```python
from build123d import *

# Parameters (mm, degrees)
F0_W     = 19.05
F0_H     = 90.4875
F1_DEPTH = 304.8
F3_W     = 12.7
F3_H     = 101.6
F4_DEPTH = 12.7
F6_DEPTH = 304.8
F8_DEPTH = 304.8


with BuildPart() as f1:
    # F0 (on Front) → F1 (new body)
    with BuildSketch(Plane.XZ):
        with Locations((9.525, 45.24375)):
            Rectangle(F0_W, F0_H)
    extrude(amount=F1_DEPTH)

    # F3 (on offset) → F4 (cut)
    with BuildSketch(Plane.XZ.offset(25.4)):
        with Locations((-1.8542, 50.8)):
            Rectangle(F3_W, F3_H)
    extrude(amount=-F4_DEPTH, mode=Mode.SUBTRACT)

    # F5 (on Front) → F6 (cut)
    with BuildSketch(Plane.XZ):
        Polygon((-2.3876, -5.089026), (26.1874, -5.089026), (26.1874, 0), (16.6624, 0), (15.604067, 4.7625), (12.429067, 4.7625), (11.370733, 0), (8.195733, 0), (7.1374, 4.7625), (-2.3876, 4.7625), align=None)
    extrude(amount=F6_DEPTH, mode=Mode.SUBTRACT)

    # F7 (on Front) → F8 (cut)
    with BuildSketch(Plane.XZ):
        Polygon((26.1874, 90.4875), (26.1874, 95.576526), (-2.3876, 95.576526), (-2.3876, 85.725), (7.1374, 85.725), (8.195733, 90.4875), (11.370733, 90.4875), (12.429067, 85.725), (15.604067, 85.725), (16.6624, 90.4875), align=None)
    extrude(amount=F8_DEPTH, mode=Mode.SUBTRACT)


solid = f1.part
```
The model under review builds one solid part; all positions refer to its coordinate system, in mm. A direction names the side the tool comes from. Round coordinates to 2 decimals unless told otherwise and drop trailing zeros. Answer as a JSON object with one key per item and string values. Group by question number.
1) For line 1 (X direction, y = -232, z = 86); line 2 (Z direction, x = 14, y = -103) (1 decimal); line 3 (X direction, y = -87.5, z = 86.5), list the stretches that pass through material, from the lowest coordinate up. Write a range as [from, to].
2) For pin 1 Ø5 at (x, y) = (4.5, -273) entering from -Z; pin 2 Ø1.6 at (x, y) = (13.5, -149.5) entering from +Z (3 decimals), all flat-tipped, find the tip position at first contact; note any pin that passes through.
3) Mouldability with a two-part tool opening along Y and no side actions: class faces 1 (the face through (4.496, -19, 45)), 2 (the face through (19.05, -150, 45)), 3 (the face through (9, 0, 46)), 4 (the face through (9, -304.8, 46)) as released by +Y, released by -Y, zero draft, split by the parting line, or undercut.
4) For faces 5 (the face through (0, -6, 45)), 6 (the face through (4, -150, 4.762)), 7 (the face through (4, -150, 85.725)), list the 3-axis set-ups (+Z, -Z, +X, -X, +Y, -Y) from which the entire face can be reached by the end or side of a thin tool; tool diameter is ignored.
Result set:
{
 "1": {"line 1": "[7.2, 12.37], [15.67, 19.05]", "line 2": "[4.8, 85.7]", "line 3": "[7.31, 12.26], [15.78, 19.05]"},
 "2": {"pin 1": "z = 4.76", "pin 2": "z = 85.725"},
 "3": {"face 1": "undercut", "face 2": "zero draft", "face 3": "released by +Y", "face 4": "released by -Y"},
 "4": {"face 5": "+Z, -Z, -X, +Y, -Y", "face 6": "-Z, -X, +Y, -Y", "face 7": "+Z, -X, +Y, -Y"}
}
